Autodesk Inventor part; units mm, degrees
ref_plane "YZ Plane" through (0, 0, 0) normal (1, 0, 0) x (0, 1, 0)
ref_plane "XZ Plane" through (0, 0, 0) normal (0, 1, 0) x (-1, 0, 0)
ref_plane "XY Plane" through (0, 0, 0) normal (0, 0, 1) x (1, 0, 0)
sketch "Sketch1" plane through (0, 0, 0) normal (0, 0, 1) x (1, 0, 0)
  line L0 (-13.5, -16) -> (13.5, -16)
  line L1 (13.5, -16) -> (13.5, 16)
  line L2 (13.5, 16) -> (-13.5, 16)
  line L3 (-13.5, 16) -> (-13.5, -16)
  line L4 (-13.5, -16) -> (13.5, 16) construction
  line L5 (13.5, -16) -> (-13.5, 16) construction
  line L6 (0, 0) -> (0, 25.8288) construction
  circle A0 centre (0, 3.5) radius 4.75
  circle A1 centre (0, 3.5) radius 3.1
  line L7 (2.1901, 1.3061) -> (-2.1901, 1.3061)
  dimension "d0" = 27
  dimension "d1" = 32
  dimension "d4" = 9.5
  dimension "d5" = 12.5
  dimension "d8" = 6.2
extrude "Extrusion1" add sketch "Sketch1" along normal blind 30 contours L3 L2 L1 L0 | A0 | A1 L7 | L7 A1
extrude "Extrusion2" add sketch "Sketch1" against normal blind 9 contours A0 | A1 L7 | L7 A1
extrude "Extrusion3" add sketch "Sketch1" against normal blind 21 contours A1 L7 picked at (0.101, 3.0658)
extrude "Extrusion4" add sketch "Sketch1" against normal blind 11.5 contours A1 L7 | L7 A1
properties part number "encoder"
Work out the finished part from the listing and answer in its coordinate system (mm). A direction names the side the tool comes from. Give positions to 0.01 mm unless a question says otherwise; leave off trailing zeros. Loops run counter-clockwise (first coordinate to the right, second up) from the corner with the lowest first, then second, coordinate; pieces in that order, holes last. Notation, with made-up numbers: (19.25, 76.25) - (26.25, 76.25) arc R5 cw to (26.25, 81.25) - close; hole circle Ø3 at (58.5, -28). An arc over 180 degrees is marked (long way). Use CSV: the item, a comma, the result in double quotes. Start each with the question number.
(1) A tool of negligible diameter and unlimited length cuts with its end or side. For faces 1 (the face through (0, 0, 30)), 2 (the face through (0, 1.306, -16)), 3 (the face through (0, 0, -9)), from which of +Z, -Z, +X, -X, +Y, -Y can it reach the whole face along a straight path? Write none if from no direction.
(2) Find section D-D, the plane y = -14. Determine the outline of the cut face in (x, z).
(3) Find the intervals of material crossed by L1, parallel to Z at x = -8.25, y = -11.5; L2, parallel to X at y = 6, z = -4; L3, parallel to X at y = 7, z = -7, in increasing order.
(4) Find section B-B, the plane x = 0. Determine the outline of the cut face in (y, z), plus the area to 3 significant figures.
(5) Find section C-C, the plane z = -15.5. Determine the outline of the cut face in (x, y), plus the area to 3 significant figures.
(6) Each of these flat-tipped pins is pushed along its axis until it touches: pin 1 (5 mm diameter, centred on y = -5, z = -10, fed in from +X); pin 2 (2 mm diameter, centred on x = 0, z = -16, fed in from -Y); pin 3 (0.5 mm diameter, centred on x = -0.5, y = 0.5, fed in from -Z); pin 4 (1.5 mm diameter, centred on x = -1, y = -6.5, fed in from -Z). Where does it stop, or does it pass through?
(7) Find section A-A, the plane y = 3.5. Determine the outline of the cut face in (x, z), plus the area to 3 significant figures.
Results found:
1,face 1,"+Z, +X, -X, +Y, -Y"
1,face 2,"-Z, +X, -X, -Y"
1,face 3,"-Z"
2,outline,"(-13.5, 0) - (13.5, 0) - (13.5, 30) - (-13.5, 30) - close"
3,L1,"0 to 30"
3,L2,"-4.04 to 4.04"
3,L3,"-3.21 to 3.21"
4,outline,"(-16, 0) - (-1.25, 0) - (-1.25, -9) - (0.4, -9) - (0.4, -11.5) - (1.31, -11.5) - (1.31, -21) - (6.6, -21) - (6.6, -9) - (8.25, -9) - (8.25, 0) - (16, 0) - (16, 30) - (-16, 30) - close"
4,area,"1,110 mm^2"
5,outline,"(-2.19, 1.31) - (2.19, 1.31) arc R3.1 ccw (long way) to start"
5,area,"27.5 mm^2"
6,pin 1,"through"
6,pin 2,"y = 1.31"
6,pin 3,"z = -11.5"
6,pin 4,"z = 0"
7,outline,"(-13.5, 0) - (-4.75, 0) - (-4.75, -9) - (-3.1, -9) - (-3.1, -21) - (3.1, -21) - (3.1, -9) - (4.75, -9) - (4.75, 0) - (13.5, 0) - (13.5, 30) - (-13.5, 30) - close"
7,area,"970 mm^2"
